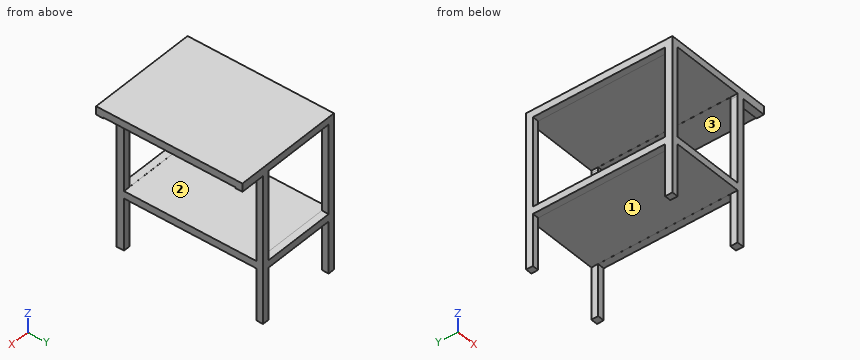
Autodesk Fusion 360 part; units mm, degrees
sketch "FrontProfile" plane through (0, 0, 0) normal (1, 0, 0) x (0, 1, 0)
  line L0 (0, 0) -> (-450, 0)
  line L1 (0, 0) -> (450, 0)
  line L2 (-450, 0) -> (-500, 0)
  line L3 (450, 0) -> (500, 0)
  line L4 (-500, 0) -> (-500, 1067)
  line L5 (500, 0) -> (500, 1066.8)
  line L6 (453.6078, 0) -> (453.6078, 1016)
  line L7 (-450, 0) -> (-450, 1016)
  line L8 (-450, 355.6) -> (453.6078, 355.6)
  line L9 (-450, 405.6) -> (453.6078, 405.6)
  line L10 (-450, 1016) -> (453.6078, 1016)
  line L11 (-500, 1067) -> (500, 1066.8)
sketch "Sketch3" plane through (0, 0, 0) normal (0, 1, 0) x (1, 0, 0)
  line L0 (0, 0) -> (-165.5064, 0)
  line L1 (-165.5064, 0) -> (-165.5064, -1016.5)
  line L2 (0, -1100) -> (-762, -1100)
  line L3 (-165.5064, 0) -> (-216.3064, 0)
  line L4 (-216.3064, 0) -> (-216.3064, -1000)
  line L5 (-762, -1100) -> (-762, 0)
  line L6 (-762, 0) -> (-711, 0)
  line L7 (-711, 0) -> (-711, -1018.0594)
  line L8 (-711, -1018.0594) -> (-165.5064, -1016.5)
  line L9 (-216.3064, -1000) -> (-216.2588, -1016.6451)
  line L10 (0, -1100) -> (0, 0)
  line L11 (-711, -356) -> (-216.3064, -356)
  line L12 (-711, 0) -> (-216.3064, 0)
  line L13 (-216.3064, -406) -> (-711, -406)
sketch "Sketch4" plane through (0, 0, 0) normal (0, 0, 1) x (1, 0, 0)
  line L0 (0, 0) -> (-762, 0)
  line L1 (0, 0) -> (0, 473.2266)
  line L2 (0, 0) -> (0, 422)
  line L3 (0, 0) -> (0, -422)
  line L4 (0, -422) -> (-750.4023, -422)
  line L5 (-750.4023, -422) -> (-762, 0)
  line L6 (0, 473.2266) -> (-750.4023, 473.2266)
  line L7 (-750.4023, 473.2266) -> (-762, 0)
  line L8 (-762, 0) -> (-762, 473.2266)
  line L9 (-762, 473.2266) -> (-750.4023, 473.2266)
  line L10 (-762, 0) -> (-762, -420)
  line L11 (-762, -420) -> (-762, -422)
  line L12 (-762, -422) -> (-697, -422)
extrude "Extrude1" add sketch "FrontProfile" against normal blind 754 contours L2 L3 L4 L5 L6 L7 L10 L11
extrude "Extrude2" add sketch "FrontProfile" against normal blind 754 contours L6 L7 L8 L9
sketch "Sketch5" plane through (0, 0, 0) normal (0, 1, 0) x (1, 0, 0)
  line L0 (-170, -1010) -> (0, -1010)
  line L1 (-170, -1010) -> (-170, 0)
sketch "Sketch6" plane through (0, 500, 0) normal (0, 1, 0) x (-1, 0, 0)
  line L0 (0, 1066.8) -> (0, 0)
  line L1 (0, 0) -> (754, 0)
  line L2 (754, 0) -> (754, 1066.8)
  line L3 (754, 1066.8) -> (0, 1066.8)
  line L4 (0, 1010) -> (170, 1010)
  line L5 (170, 1010) -> (170, 0)
  line L6 (170, 0) -> (0, 0)
  line L7 (0, 0) -> (0, 1010)
extrude "Extrude3" cut sketch "Sketch6" against normal blind 1000 contours L0 L1 L4 L5 L6 L7
extrude "Extrude4" cut sketch "Sketch3" along normal blind 600 contours L4 L7 L8 L9 L13
extrude "Extrude5" cut sketch "Sketch3" against normal blind 700 contours L4 L7 L8 L9 L13
extrude "Extrude6" cut sketch "Sketch3" against normal blind 650 contours L4 L7 L11 L12
extrude "Extrude7" cut sketch "Sketch3" along normal blind 600 contours L4 L7 L11 L12
Could you check a few things on this model? Use its own coordinates, in mm. Face numbers are marked on the shaded views. Give positions to 0.01 mm unless a question says otherwise; leave off trailing zeros. Loops run counter-clockwise (first coordinate to the right, second up) from the corner with the lowest first, then second, coordinate; pieces in that order, holes last. Notation, with made-up numbers: (9, 82) -> (28, 82) arc R35 cw to (28, 118) -> close; hole circle Ø11 at (66.25, 41). An arc over 180 degrees is marked (long way). Answer as CSV lines item,"result". Start each with the question number.
(1) If we section it at A-A on z = 519: Write out the boundary of the cut face in (x, y), then the cut area to 3 significant figures.
(2) If we section it at D-D on x = -140: Write out the boundary of the cut face in (y, z), then the cut area to 3 significant figures.
(3) We'd pull the mould along Z, two halves only. Please class the marked faces 1, 2 and 3: released by +Z, released by -Z, zero draft, split by the parting line, or undercut.
(4) If we section it at C-C on x = -634: Write out the boundary of the cut face in (y, z), then the cut area to 3 significant figures.
(5) If we section it at B-B on y = 332: Write out the boundary of the cut face in (x, z).
(6) I need wall thicknesses on probe 1 along Z at (x, y) = (-682, -282); probe 2 along Z at (x, y) = (-723, 274); probe 3 along Z at (x, y) = (-106.5, 216). Which ranges of each line are inside material? Lowest first, please.
(7) I'm going to push flat-ended pins straight in: pin 1 Ø10 at (x, y) = (-400, -196) entering from +Z; pin 2 Ø12 at (x, y) = (-474, -330) entering from +Z; pin 3 Ø6 at (x, y) = (-276.5, 397.5) entering from +Z. Where does each tip first touch, or does it pass through?
Computed:
1,outline,"(-754, -500) -> (-711, -500) -> (-711, -450) -> (-754, -450) -> close; (-754, 453.61) -> (-711, 453.61) -> (-711, 500) -> (-754, 500) -> close; (-216.31, -500) -> (-170, -500) -> (-170, -450) -> (-216.31, -450) -> close; (-216.31, 453.61) -> (-170, 453.61) -> (-170, 500) -> (-216.31, 500) -> close"
1,area,"8,610 mm2"
2,outline,"(-500, 1010) -> (-450, 1010) -> (-450, 1016) -> (453.61, 1016) -> (453.61, 1010) -> (500, 1010) -> (500, 1066.8) -> (-500, 1067) -> close"
2,area,"51,500 mm2"
3,face 1,"released by -Z"
3,face 2,"undercut"
3,face 3,"undercut"
4,outline,"(-500, 356) -> (500, 356) -> (500, 406) -> (453.61, 406) -> (453.61, 405.6) -> (-450, 405.6) -> (-450, 406) -> (-500, 406) -> close; (-500, 1017.84) -> (500, 1017.84) -> (500, 1066.8) -> (-500, 1067) -> close"
4,area,"98,700 mm2"
5,outline,"(-754, 355.6) -> (-711, 355.6) -> (-711, 356) -> (-216.31, 356) -> (-216.31, 355.6) -> (-170, 355.6) -> (-170, 405.6) -> (-754, 405.6) -> close; (-754, 1016) -> (-711, 1016) -> (-711, 1018.06) -> (-216.26, 1016.65) -> (-216.26, 1016) -> (0, 1016) -> (0, 1066.83) -> (-754, 1066.83) -> close"
6,probe 1,"z = 356 to 405.6, 1017.98 to 1066.96"
6,probe 2,"z = 355.6 to 405.6, 1016 to 1066.85"
6,probe 3,"z = 1016 to 1066.86"
7,pin 1,"stops at z = 1066.94"
7,pin 2,"stops at z = 1066.97"
7,pin 3,"stops at z = 1066.82"
